Build history of the part. All positions in model axes, mm. A direction names the side the tool comes from. Round coordinates to 2 decimals unless told otherwise and drop trailing zeros. Write each loop counter-clockwise with the first axis right and the second up, starting at its lowest first coordinate (ties: lowest second). Pieces come first, ordered by that corner, then holes. Notation, with made-up numbers: (18.5, 44) -> (30.5, 44) arc R36 cw to (30.5, 78) -> close; hole circle Ø11 at (-19.75, -6.5). An arc over 180 degrees is marked (long way). One line per question, with ' | ' between items.
Autodesk Inventor part; units mm, degrees
ref_plane "YZ Plane" through (0, 0, 0) normal (1, 0, 0) x (0, 1, 0)
ref_plane "XZ Plane" through (0, 0, 0) normal (0, 1, 0) x (-1, 0, 0)
ref_plane "XY Plane" through (0, 0, 0) normal (0, 0, 1) x (1, 0, 0)
sketch "Sketch1" plane through (0, 0, 0) normal (0, 0, 1) x (1, 0, 0)
  line L0 (7.62, 0) -> (60.96, 0)
  line L1 (68.58, 7.62) -> (68.58, 35.56)
  line L2 (60.96, 43.18) -> (7.62, 43.18)
  line L3 (0, 35.56) -> (0, 7.62)
  arc A0 (7.62, 43.18) -> (0, 35.56) centre (7.62, 35.56) ccw
  arc A1 (0, 7.62) -> (7.62, 0) centre (7.62, 7.62) ccw
  arc A2 (60.96, 0) -> (68.58, 7.62) centre (60.96, 7.62) ccw
  arc A3 (68.58, 35.56) -> (60.96, 43.18) centre (60.96, 35.56) ccw
  point P0 (0, 0)
  point P1 (68.58, 43.18)
  point P2 (68.58, 0)
  point P3 (0, 43.18)
  dimension "d0" = 68.58
  dimension "d1" = 43.18
  dimension "d2" = 7.62
extrude "Extrusion1" add sketch "Sketch1" along normal blind 25.4
sketch "Sketch2" plane through (0, 0, 25.4) normal (0, 0, 1) x (1, 0, 0)
  line L0 (-0.635, -3.81) -> (69.215, -3.81)
  line L1 (72.39, -0.635) -> (72.39, 43.815)
  line L2 (69.215, 46.99) -> (-0.635, 46.99)
  line L3 (-3.81, 43.815) -> (-3.81, -0.635)
  arc A0 (-0.635, 46.99) -> (-3.81, 43.815) centre (-0.635, 43.815) ccw
  arc A1 (-3.81, -0.635) -> (-0.635, -3.81) centre (-0.635, -0.635) ccw
  arc A2 (69.215, -3.81) -> (72.39, -0.635) centre (69.215, -0.635) ccw
  arc A3 (72.39, 43.815) -> (69.215, 46.99) centre (69.215, 43.815) ccw
  line L4 (60.96, 43.18) -> (7.62, 43.18) construction
  line L5 (0, 35.56) -> (0, 7.62) construction
  point P0 (0, 0)
  point P1 (72.39, 46.99)
  point P2 (72.39, -3.81)
  point P3 (-3.81, 46.99)
  point P4 (34.29, 46.99)
  point P5 (34.29, 43.18)
  point P6 (-3.81, 21.59)
  point P7 (0, 21.59)
  dimension "d5" = 76.2
  dimension "d6" = 50.8
  dimension "d7" = 3.175
extrude "Extrusion2" add sketch "Sketch2" along normal blind 12.7
fillet "Fillet1" radius 3.175 8 edges at (-2.8801, 46.0601, 38.1) (-3.81, 21.59, 38.1) (-2.8801, -2.8801, 38.1) (34.29, -3.81, 38.1) (71.4601, -2.8801, 38.1) (72.39, 21.59, 38.1) (71.4601, 46.0601, 38.1) (34.29, 46.99, 38.1)
sketch "Sketch3" plane through (0, 0, 38.1) normal (0, 0, 1) x (1, 0, 0)
  line L0 (69.215, 46.99) -> (-0.635, 46.99) construction
  line L1 (69.215, 46.99) -> (-0.635, 46.99) construction
  line L2 (-3.81, 43.815) -> (-3.81, -0.635) construction
  line L3 (-3.81, 43.815) -> (-3.81, -0.635) construction
  circle A0 centre (34.29, 21.59) radius 8.75
  circle A1 centre (34.29, 21.59) radius 19 construction
  circle A2 centre (20.855, 35.025) radius 2.25
  circle A3 centre (47.725, 35.025) radius 2.25
  circle A4 centre (15.29, 21.59) radius 2.25
  circle A5 centre (53.29, 21.59) radius 2.25
  circle A6 centre (20.855, 8.155) radius 2.25
  circle A7 centre (47.725, 8.155) radius 2.25
  line L4 (20.855, 35.025) -> (34.29, 21.59) construction
  line L5 (34.29, 21.59) -> (15.29, 21.59) construction
  point P0 (0, 0)
  point P1 (34.29, 46.99)
  point P2 (-3.81, 21.59)
  point P3 (-3.81, 21.59)
  dimension "d11" = 17.5
  dimension "d14" = 4.5
  dimension "d15" = 38
  dimension "d16" = 45
extrude "Extrusion3" cut sketch "Sketch3" against normal up to surface (38.1 mm away)
chamfer "Chamfer1" distance 1.27 angle 45 6 edges at (45.475, 35.025, 0) (18.605, 35.025, 0) (13.04, 21.59, 0) (51.04, 21.59, 0) (45.475, 8.155, 0) (18.605, 8.155, 0)
properties part number "2x3_Spacer_Rear"
(1) Slice it at B-B (y = 21.59). Write the cut outline in (x, z) (3 decimals).
Calculated:
outline: (-3.81, 25.4) -> (0, 25.4) -> (0, 0) -> (11.77, 0) -> (13.04, 1.27) -> (13.04, 38.1) -> (-0.635, 38.1) arc R3.175 ccw to (-3.81, 34.925) -> close; (17.54, 1.27) -> (18.81, 0) -> (25.54, 0) -> (25.54, 38.1) -> (17.54, 38.1) -> close; (43.04, 0) -> (49.77, 0) -> (51.04, 1.27) -> (51.04, 38.1) -> (43.04, 38.1) -> close; (55.54, 1.27) -> (56.81, 0) -> (68.58, 0) -> (68.58, 25.4) -> (72.39, 25.4) -> (72.39, 34.925) arc R3.175 ccw to (69.215, 38.1) -> (55.54, 38.1) -> close
(2) Mould opens along X. For faces 4 (the cylindrical face through (71.48, -2.86, 30.1)), 5 (the flat face through (26, 27, 0)), 6 (the cylindrical face through (45.939, 33.656, 19.943)) say: pulls with the +X half, pulls with the -X half, needs draft (parallel to the pull), parting line crosses it, or undercut.
Calculated:
face 4: pulls with the +X half | face 5: needs draft | face 6: undercut
(3) Wall check: line 1 (X direction, y = 35, z = 33); line 2 (X direction, y = 10, z = 31); line 3 (Y direction, x = 34, z = 25). Give the ranges that are in metal, low to high. Write a range as from..to.
Calculated:
line 1: -3.81..18.61, 23.1..45.48, 49.97..72.39 | line 2: -3.81..19.57, 22.14..46.44, 49.01..72.39 | line 3: 0..12.84, 30.34..43.18
(4) Slice it at C-C (z = 34). Write the cut outline in (x, y) (3 decimals).
Calculated:
outline: (-3.81, -0.635) arc R3.175 ccw to (-0.635, -3.81) -> (69.215, -3.81) arc R3.175 ccw to (72.39, -0.635) -> (72.39, 43.815) arc R3.175 ccw to (69.215, 46.99) -> (-0.635, 46.99) arc R3.175 ccw to (-3.81, 43.815) -> close; hole circle Ø4.5 at (15.29, 21.59); hole circle Ø4.5 at (20.855, 8.155); hole circle Ø4.5 at (20.855, 35.025); hole circle Ø17.5 at (34.29, 21.59); hole circle Ø4.5 at (47.725, 8.155); hole circle Ø4.5 at (47.725, 35.025); hole circle Ø4.5 at (53.29, 21.59)
(5) Slice it at A-A (x = 15.29). Write the cut outline in (y, z) (3 decimals), then the cut area to 3 significant figures.
Calculated:
outline: (-3.81, 25.4) -> (0, 25.4) -> (0, 0) -> (18.07, 0) -> (19.34, 1.27) -> (19.34, 38.1) -> (-0.635, 38.1) arc R3.175 ccw to (-3.81, 34.925) -> close; (23.84, 1.27) -> (25.11, 0) -> (43.18, 0) -> (43.18, 25.4) -> (46.99, 25.4) -> (46.99, 34.925) arc R3.175 ccw to (43.815, 38.1) -> (23.84, 38.1) -> close | area: 1,560 mm2
(6) Slice it at D-D (x = 32). Write the cut outline in (y, z) (3 decimals), then the cut area to 3 significant figures.
Calculated:
outline: (-3.81, 25.4) -> (0, 25.4) -> (0, 0) -> (13.145, 0) -> (13.145, 38.1) -> (-0.635, 38.1) arc R3.175 ccw to (-3.81, 34.925) -> close; (30.035, 0) -> (43.18, 0) -> (43.18, 25.4) -> (46.99, 25.4) -> (46.99, 34.925) arc R3.175 ccw to (43.815, 38.1) -> (30.035, 38.1) -> close | area: 1,090 mm2
(7) Drop flat-ended pins along their axis: pin 1 (7.5 mm diameter, centred on x = 33, z = 9, fed in from -Y); pin 2 (6 mm diameter, centred on x = 20.855, y = 8.155, fed in from -Z); pin 3 (8 mm diameter, centred on y = 36, z = 12.5, fed in from -X). Give the stop position or say it passes through.
Calculated:
pin 1: y = 0 | pin 2: z = 0.52 | pin 3: x = 0
(8) 3-axis set-ups, long thin cutter, end or side, ignore diameter. For faces 1 (the flat face through (0, 22, 13)), 2 (the cylindrical face through (66.407, 2.291, 12.522)), 3 (the flat face through (34, 0, 13)): which of +Z, -Z, +X, -X, +Y, -Y reach the whole face in a straight line?
Calculated:
face 1: -Z, -X, +Y, -Y | face 2: -Z, +X, -Y | face 3: -Z, +X, -X, -Y
